```python
from build123d import *

# Parameters (mm, degrees)
F0_R     = 10.65
F1_DEPTH = 10
F2_R     = 11.15
F2_R_2   = 10.65
F3_DEPTH = 1
F7_R     = 3.15
F8_DEPTH = 27.57


with BuildPart() as f1:
    # F0 (on Top) → F1 (new body)
    with BuildSketch(Plane.XY):
        Circle(F0_R)
    extrude(amount=F1_DEPTH)

    # F2 (on face) → F3 (join)
    with BuildSketch(Plane.XY.offset(10)):
        Circle(F2_R)
        Circle(F2_R_2, mode=Mode.SUBTRACT)
        Circle(F2_R_2)
    extrude(amount=F3_DEPTH)

    # F7 (on face) → F8 (cut)
    with BuildSketch(Plane(origin=(0, 16.688987, 17.823191), x_dir=(1, 0, 0), z_dir=(0, 0.6835, 0.729951))):
        with Locations((0, -4.124223)):
            Circle(F7_R)
    extrude(amount=-F8_DEPTH, mode=Mode.SUBTRACT)


solid = f1.part
```
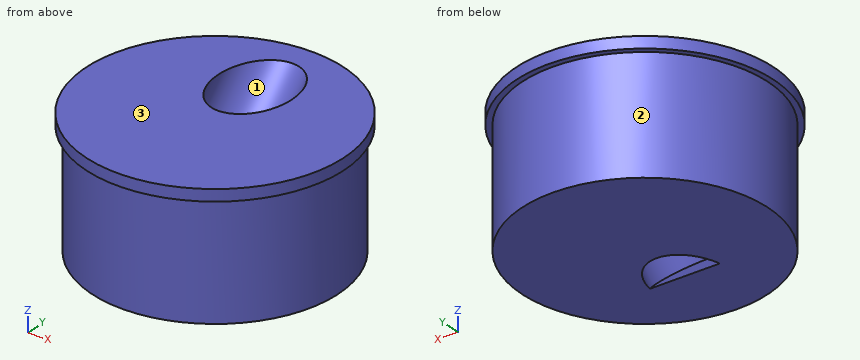
Source: CAD feature listing. Evaluate the final solid. Frame: model axes, mm. Face numbers are marked on the shaded views. Give positions to 0.01 mm unless a question says otherwise; leave off trailing zeros. Loops run counter-clockwise (first coordinate to the right, second up) from the corner with the lowest first, then second, coordinate; pieces in that order, holes last. Notation, with made-up numbers: (88.25, 78) -> (125.25, 78) arc R23 ccw to (125.25, 112) -> close; hole circle Ø5 at (-7, 50.5). An arc over 180 degrees is marked (long way). Put each result on its own line as item: value. Start each with the question number.
1) Material intervals for probe 1 along X at (y, z) = (2.5, 8.25); probe 2 along X at (y, z) = (1.25, 6.5); probe 3 along Y at (x, z) = (1.5, 5), sorted ascending.
2) Cut plane A-A (x = 1.25). Return loops of the section in (y, z), then the cut area to 3 significant figures.
3) Cut plane B-B (x = -7). Return loops of the section in (y, z).
4) Draft query along Y for the marked faces 1, 2 and 3. Return one class per face: released by +Y, released by -Y, zero draft, split by the parting line, or undercut.
5) Contact query for flat-ended pins moving along their axis: P1, Ø5, axis at x = -1, z = 4, coming from the -Y side; P2, Ø3, axis at x = -6.5, z = 6, coming from the -Y side; P3, Ø2, axis at y = -0.5, z = 3.5, coming from the +X side. Output: stop coordinate, or through.
Results are:
1. probe 1: x = -10.35 to -3.13, 3.13 to 10.35
1. probe 2: x = -10.58 to -3.09, 3.09 to 10.58
1. probe 3: y = -10.54 to -4.76, 2.83 to 10.54
2. outline: (-11.08, 10) -> (-10.58, 10) -> (-10.58, 0) -> (-4.61, 0) -> (-7.28, 2.49) -> (0.69, 11) -> (-11.08, 11) -> close; (-1.69, 0) -> (10.58, 0) -> (10.58, 10) -> (11.08, 10) -> (11.08, 11) -> (8.61, 11) -> close
2. area: 153 mm2
3. outline: (-8.68, 10) -> (-8.03, 10) -> (-8.03, 0) -> (8.03, 0) -> (8.03, 10) -> (8.68, 10) -> (8.68, 11) -> (-8.68, 11) -> close
4. face 1: undercut
4. face 2: split by the parting line
4. face 3: zero draft
5. P1: stops at y = -10.65
5. P2: stops at y = -9.4
5. P3: stops at x = 10.65
